CAD build for the part. Positions are in the model's coordinates, mm. A direction names the side the tool comes from. Give positions to 0.01 mm unless a question says otherwise; leave off trailing zeros. Write each loop counter-clockwise with the first axis right and the second up, starting at its lowest first coordinate (ties: lowest second). Pieces come first, ordered by that corner, then holes. Notation, with made-up numbers: (55.5, -10.5) - (76.5, -10.5) arc R14 cw to (76.5, 11.5) - close; hole circle Ø8 at (71.25, 60.5). An arc over 180 degrees is marked (long way). Write item = value, one per line. Start each with the question number.
```python
from build123d import *

# Parameters (mm, degrees)
F0_W     = 50
F0_H     = 50
F1_DEPTH = 20
F1_TAPER = 10
F4_DEPTH = 2.5
F5_W     = 42.9469207717
F5_H     = 33.9469207717
F6_DEPTH = 10


with BuildPart() as f1:
    # F0 (on Top) → F1 (new body)
    with BuildSketch(Plane.XY):
        Rectangle(F0_W, F0_H)
    extrude(amount=F1_DEPTH, taper=F1_TAPER)

    # F3 (on face) → F4 (cut)
    with BuildSketch(Plane(origin=(0, 24.2461577598, 4.2752517916), x_dir=(-1, 0, 0), z_dir=(0, 0.984807753, 0.1736481777))):
        with BuildLine():
            ThreePointArc((-62.6127916525, 12.0467824013), (-65.1076142535, 12.9570129346), (-67.6967318406, 13.5478847947))
            Line((-67.6967318406, 13.5478847947), (-67.6967318406, 1.7008224913))
            Line((-67.6967318406, 1.7008224913), (-64.9974017565, 0.6510827954))
            Line((-64.9974017565, 0.6510827954), (-64.9974017565, 10.8966148214))
            ThreePointArc((-64.9974017565, 10.8966148214), (-64.4272854823, 11.4667310956), (-63.8571692081, 10.8966148214))
            Line((-63.8571692081, 10.8966148214), (-63.8571692081, 6.5746134929))
            ThreePointArc((-63.8571692081, 6.5746134929), (-63.1556576777, 6.2062071738), (-62.36370085, 6.1807901262))
            ThreePointArc((-62.36370085, 6.1807901262), (-61.4973256009, 6.5898476466), (-60.9304969783, 7.3622720376))
            ThreePointArc((-60.9304969783, 7.3622720376), (-60.8139105128, 8.6329221267), (-60.9304969783, 9.9035722157))
            ThreePointArc((-60.9304969783, 9.9035722157), (-61.4992901353, 11.1889594143), (-62.6127916525, 12.0467824013))
        make_face()
        with BuildLine():
            Line((-59.852306272, 4.1264343026), (-64.3468709521, 2.5074238792))
            Line((-64.3468709521, 2.5074238792), (-64.3468709521, 0.8903192669))
            Line((-64.3468709521, 0.8903192669), (-59.1967386775, 2.745475089))
            ThreePointArc((-59.1967386775, 2.745475089), (-58.3600263338, 3.0909475212), (-57.5693056666, 3.5316283287))
            ThreePointArc((-57.5693056666, 3.5316283287), (-57.2106825124, 3.8266438133), (-57.1279449174, 4.2835893169))
            ThreePointArc((-57.1279449174, 4.2835893169), (-57.2731405563, 4.626683197), (-57.5693056666, 4.8526951689))
            ThreePointArc((-57.5693056666, 4.8526951689), (-59.1391575222, 5.4515460975), (-60.8064195051, 5.6596200345))
            ThreePointArc((-60.8064195051, 5.6596200345), (-62.3430133295, 5.6105588901), (-63.8571692081, 5.3443643137))
            Line((-63.8571692081, 5.3443643137), (-64.3733816954, 5.1584167399))
            Line((-64.3733816954, 5.1584167399), (-64.3733816954, 3.567821243))
            Line((-64.3733816954, 3.567821243), (-61.5377031577, 4.5892756967))
            ThreePointArc((-61.5377031577, 4.5892756967), (-61.4484140803, 4.623308608), (-61.3579327635, 4.6540317215))
            ThreePointArc((-61.3579327635, 4.6540317215), (-60.7215197269, 4.7724043893), (-60.0756078839, 4.7296079809))
            ThreePointArc((-60.0756078839, 4.7296079809), (-59.8276638338, 4.6512158498), (-59.6342471347, 4.4774011246))
            ThreePointArc((-59.6342471347, 4.4774011246), (-59.607836679, 4.389638385), (-59.6342471347, 4.3018756454))
            ThreePointArc((-59.6342471347, 4.3018756454), (-59.7293419591, 4.1968352348), (-59.852306272, 4.1264343026))
        make_face()
        with BuildLine():
            Line((-61.5377031577, 4.5892756967), (-61.3579327635, 4.6540317215))
            ThreePointArc((-61.3579327635, 4.6540317215), (-61.4484140803, 4.623308608), (-61.5377031577, 4.5892756967))
        make_face()
        with BuildLine():
            Line((-71.3693953118, 3.7232309117), (-68.2338687675, 4.8526951689))
            Line((-68.2338687675, 4.8526951689), (-68.2338687675, 6.3986412263))
            Line((-68.2338687675, 6.3986412263), (-72.8589746057, 4.7326078963))
            ThreePointArc((-72.8589746057, 4.7326078963), (-73.3660543121, 4.4190102256), (-73.7959157464, 4.0058607672))
            ThreePointArc((-73.7959157464, 4.0058607672), (-73.8489158308, 3.7221286407), (-73.7959157464, 3.4383965142))
            ThreePointArc((-73.7959157464, 3.4383965142), (-73.5719055484, 3.0819711924), (-73.2075114709, 2.8711714412))
            ThreePointArc((-73.2075114709, 2.8711714412), (-72.698935386, 2.6276316569), (-72.151396822, 2.4928622925))
            ThreePointArc((-72.151396822, 2.4928622925), (-71.0199458053, 2.2564276603), (-69.8657767964, 2.1933670766))
            ThreePointArc((-69.8657767964, 2.1933670766), (-69.0466795364, 2.2155081429), (-68.2338687675, 2.3191865022))
            Line((-68.2338687675, 2.3191865022), (-68.2338687675, 3.7681726435))
            ThreePointArc((-68.2338687675, 3.7681726435), (-68.7127832674, 3.5843780991), (-69.2045442964, 3.4383965142))
            ThreePointArc((-69.2045442964, 3.4383965142), (-70.2705361783, 3.1526989385), (-71.3693953118, 3.2550239211))
            ThreePointArc((-71.3693953118, 3.2550239211), (-71.4727799338, 3.4891274164), (-71.3693953118, 3.7232309117))
        make_face()
        with BuildLine():
            Line((-8.8550038247, 8.9253647507), (-18.3714963496, 8.9253647507))
            Line((-18.3714963496, 8.9253647507), (-18.3714963496, 8.0944637033))
            Line((-18.3714963496, 8.0944637033), (-9.6104234449, 8.0944637033))
            ThreePointArc((-9.6104234449, 8.0944637033), (-8.2918347743, 6.7758750328), (-9.6104234449, 5.4572863622))
            Line((-9.6104234449, 5.4572863622), (-16.3685619547, 5.4572863622))
            ThreePointArc((-16.3685619547, 5.4572863622), (-17.7848504476, 4.8706404602), (-18.3714963496, 3.4543519673))
            Line((-18.3714963496, 3.4543519673), (-18.3714963496, 0.8903192669))
            Line((-18.3714963496, 0.8903192669), (-16.6691035906, 0.8903192669))
            Line((-16.6691035906, 0.8903192669), (-16.6691035906, 3.2509914089))
            ThreePointArc((-16.6691035906, 3.2509914089), (-16.3194164791, 4.0952107761), (-15.475197112, 4.4448978876))
            Line((-15.475197112, 4.4448978876), (-8.8550038247, 4.4448978876))
            ThreePointArc((-8.8550038247, 4.4448978876), (-6.6147703931, 6.6851313191), (-8.8550038247, 8.9253647507))
        make_face()
        with BuildLine():
            Line((6.6308597895, 8.0305831634), (6.6308597895, 8.8359827707))
            Line((6.6308597895, 8.8359827707), (1.2028706223, 8.8359827707))
            ThreePointArc((1.2028706223, 8.8359827707), (-0.2622622882, 8.2291048484), (-0.8691402105, 6.7639719379))
            Line((-0.8691402105, 6.7639719379), (-0.8691402105, 2.7997734057))
            ThreePointArc((-0.8691402105, 2.7997734057), (-1.1781523708, 2.0537520573), (-1.9241737192, 1.744739897))
            Line((-1.9241737192, 1.744739897), (-6.9461943019, 1.744739897))
            Line((-6.9461943019, 1.744739897), (-6.9461943019, 0.9224587447))
            Line((-6.9461943019, 0.9224587447), (-1.1303118512, 0.9224587447))
            ThreePointArc((-1.1303118512, 0.9224587447), (-0.9994251278, 0.9268988758), (-0.8691402105, 0.9401988537))
            ThreePointArc((-0.8691402105, 0.9401988537), (0.324782393, 1.5838337022), (0.8010555712, 2.8538261671))
            Line((0.8010555712, 2.8538261671), (0.8010555712, 6.7639719379))
            ThreePointArc((0.8010555712, 6.7639719379), (1.17203741, 7.6596013245), (2.0676667967, 8.0305831634))
            Line((2.0676667967, 8.0305831634), (6.6308597895, 8.0305831634))
        make_face()
        with BuildLine():
            Line((-0.8691402105, 0.9224587447), (-0.8691402105, 0.9401988537))
            ThreePointArc((-0.8691402105, 0.9401988537), (-0.9994251278, 0.9268988758), (-1.1303118512, 0.9224587447))
            Line((-1.1303118512, 0.9224587447), (-0.8691402105, 0.9224587447))
        make_face()
        with BuildLine():
            Line((16.1497702226, 8.7293623708), (6.2916715828, 2.7671895852))
            ThreePointArc((6.2916715828, 2.7671895852), (6.0312638327, 2.1103408421), (6.5940157184, 1.6830554777))
            Line((6.5940157184, 1.6830554777), (15.6298977944, 1.6830554777))
            Line((15.6298977944, 1.6830554777), (15.6298977944, 0.8854835551))
            Line((15.6298977944, 0.8854835551), (17.3096715009, 0.8854835551))
            Line((17.3096715009, 0.8854835551), (17.3096715009, 1.6830554777))
            Line((17.3096715009, 1.6830554777), (18.9957390394, 1.6830554777))
            Line((18.9957390394, 1.6830554777), (18.9957390394, 2.5790360808))
            Line((18.9957390394, 2.5790360808), (17.3096715009, 2.5790360808))
            Line((17.3096715009, 2.5790360808), (17.3096715009, 8.4309516424))
            ThreePointArc((17.3096715009, 8.4309516424), (16.7924307072, 8.8239057157), (16.1497702226, 8.7293623708))
        make_face()
        with BuildLine():
            ThreePointArc((15.6298977944, 2.7664388472), (15.5851471152, 2.650295301), (15.4830977637, 2.5790360808))
            Line((15.4830977637, 2.5790360808), (8.2873353154, 2.5790360808))
            ThreePointArc((8.2873353154, 2.5790360808), (8.2396752723, 2.5724973144), (8.1920152292, 2.5790360808))
            ThreePointArc((8.1920152292, 2.5790360808), (8.0660077379, 2.7154691755), (8.1312813761, 2.8893404766))
            ThreePointArc((8.1312813761, 2.8893404766), (8.1482094403, 2.900951867), (8.1663682644, 2.9105247899))
            Line((8.1663682644, 2.9105247899), (15.2921648042, 7.212847216))
            ThreePointArc((15.2921648042, 7.212847216), (15.4818399907, 7.2366014749), (15.6298977944, 7.1156889945))
            Line((15.6298977944, 7.1156889945), (15.6298977944, 2.7966582224))
            ThreePointArc((15.6298977944, 2.7966582224), (15.6304347873, 2.7815485348), (15.6298977944, 2.7664388472))
        make_face(mode=Mode.SUBTRACT)
    extrude(amount=-F4_DEPTH, mode=Mode.SUBTRACT)

    # F5 (on face) → F6 (cut)
    with BuildSketch(Plane.XY.offset(20)):
        Polygon((-21.4734603858, 12.4734603858), (-40, 12.4734603858), (-40, -37.5265396142), (40, -37.5265396142), (40, 12.4734603858), (21.4734603858, 12.4734603858), (21.4734603858, -21.4734603858), (-21.4734603858, -21.4734603858), align=None)
        with Locations((0, -4.5)):
            Rectangle(F5_W, F5_H)
    extrude(amount=-F6_DEPTH, mode=Mode.SUBTRACT)


solid = f1.part
```
1. Cut at C-C (z = 18.25). Give the cut face in (x, y).
2. Tool access for faces 1 (the flat face through (-11.679, 22.159, 9.016)), 2 (the flat face through (-12.74, 23.49, 8.57)), 3 (the flat face through (-18.16, 22.58, 6.6)): list every direction of +Z, -Z, +X, -X, +Y, -Y with a clear straight run to the whole face (end or side of a thin tool).
3. Wall check: line 1 along Z through (x, y) = (10.5, -17); line 2 along X through (y, z) = (3, 4.25); line 3 along X through (y, z) = (-4, 7). Give the ranges that are in metal, low to high.
4. Cut at A-A (y = 15.5). Give the cut face in (x, z).
5. Mould opens along Z. For faces 4 (the flat face through (-11.05, 22.74, 5.72)), 5 (the flat face through (24.045, 0.35, 5.416)), 6 (the flat face through (12.21, 22.26, 8.44)) say: +Z half, -Z half, draft (parallel to the pull), parting line (faces both ways), or undercut.
6. Pin check, flat tips, straight feed: pin 1 Ø4 at (y, z) = (-6.5, 3) entering from -X; pin 2 Ø18 at (x, y) = (10, 0) entering from +Z; pin 3 Ø10 at (x, z) = (1, 13) entering from +Y. Stop position of each tip, or through.
7. Cut at B-B (x = -13). Give the cut face in (y, z).
Output:
q1.outline = (-21.78, 12.47) - (21.78, 12.47) - (21.78, 21.78) - (-21.78, 21.78) - close
q2.face_1 = none
q2.face_2 = +Z, +X, -X, +Y
q2.face_3 = +Y
q3.line_1 = 0 to 10
q3.line_2 = -24.25 to 24.25
q3.line_3 = -23.77 to 23.77
q4.outline = (-25, 0) - (25, 0) - (21.47, 20) - (-21.47, 20) - close
q5.face_4 = undercut
q5.face_5 = +Z half
q5.face_6 = undercut
q6.pin_1 = -24.82
q6.pin_2 = 10
q6.pin_3 = 23.59
q7.outline = (-25, 0) - (25, 0) - (23.95, 5.93) - (21.49, 5.5) - (21.34, 6.38) - (23.8, 6.82) - (23.23, 10.02) - (20.77, 9.58) - (20.6, 10.56) - (23.06, 11) - (21.47, 20) - (12.47, 20) - (12.47, 10) - (-23.24, 10) - close
